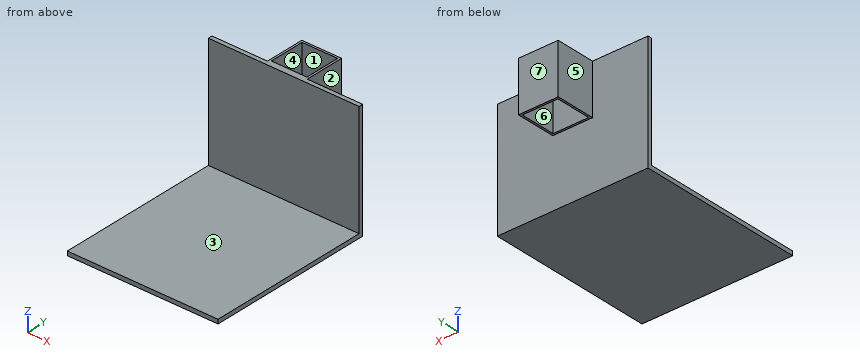
```python
from build123d import *

# Parameters (mm, degrees)
F0_W     = 60.325
F0_H     = 60.325
F0_W_2   = 53.975
F0_H_2   = 53.975
F1_DEPTH = 76.2
F3_DEPTH = 114.3


with BuildPart() as f1:
    # F0 (on Top) → F1 (new body)
    with BuildSketch(Plane.XY):
        Rectangle(F0_W, F0_H)
        Rectangle(F0_W_2, F0_H_2, mode=Mode.SUBTRACT)
    extrude(amount=F1_DEPTH)

    # F2 (on Right) → F3 (join, symmetric)
    with BuildSketch(Plane.YZ):
        Polygon((-30.1625, -101.6), (-30.1625, 76.2), (-36.5125, 76.2), (-36.5125, -95.25), (-284.1625, -95.25), (-284.1625, -101.6), align=None)
    extrude(amount=F3_DEPTH, both=True)


solid = f1.part
```
Check sheet for the modelled part. Datum: model origin and axes. Units: mm. Face numbers are marked on the shaded views. A direction names the side the tool comes from. Give positions to 0.01 mm unless a question says otherwise; leave off trailing zeros. Order: outer loops, then holes, each group sorted by start corner. A loop starts at its lowest first (then second) coordinate and runs counter-clockwise, first axis right, second up. Notation, with made-up numbers: M 23.25,81 L 68.25,81 A12 cw 68.25,94 Z; hole C -7,34 d2. An arc over 180 degrees is marked long. Answer in a Markdown table with one row per item. Add a question column.
Q1. Thickness scan on L1, parallel to X at y = -11.5, z = 14.5; L2, parallel to Y at x = -1, z = 1; L3, parallel to Z at x = 31.5, y = -67.5. Record the ranges inside material, lowest first.
Q2. Sectioned sample at A-A, the plane x = -6.5. Record the boundary of the cut face in (y, z), and give its area (3 significant figures).
Q3. Gauge pin test, flat ends, axial feed: pin 1 Ø16 at (y, z) = (-3.5, 33.5) entering from +X; pin 2 Ø1.5 at (x, z) = (83.5, 47.5) entering from -Y; pin 3 Ø2 at (y, z) = (-18.5, 16) entering from -X; pin 4 Ø18 at (x, y) = (6.5, -14.5) entering from -Z. Record the tip position at first contact, or that the pin passes through.
Q4. Sectioned sample at D-D, the plane x = 92.5. Record the boundary of the cut face in (y, z).
Q5. Access from +Z, -Z, +X, -X, +Y, -Y to the whole of each face (thin tool, end or side, straight path). Record for the marked faces 1, 2 and 3.
Q6. Release check for a two-part mould opening along Y. For the marked faces 4, 5, 6 and 7 record: released by +Y, released by -Y, zero draft, split by the parting line, or undercut.
Q7. Sectioned sample at C-C, the plane z = 36. Record the boundary of the cut face in (x, y), and give its area (3 significant figures).
Q8. Sectioned sample at B-B, the plane y = -12. Record the boundary of the cut face in (x, z).
Verdict:
| question | item | result |
|---|---|---|
| 1 | L1 | -30.16 to -26.99, 26.99 to 30.16 |
| 1 | L2 | -36.51 to -26.99, 26.99 to 30.16 |
| 1 | L3 | -101.6 to -95.25 |
| 2 | outline | M -284.16,-101.6 L -30.16,-101.6 L -30.16,0 L -26.99,0 L -26.99,76.2 L -36.51,76.2 L -36.51,-95.25 L -284.16,-95.25 Z; M 26.99,0 L 30.16,0 L 30.16,76.2 L 26.99,76.2 Z |
| 2 | area | 3,190 mm² |
| 3 | pin 1 | x = 30.16 |
| 3 | pin 2 | y = -36.51 |
| 3 | pin 3 | x = -30.16 |
| 3 | pin 4 | through |
| 4 | outline | M -284.16,-101.6 L -30.16,-101.6 L -30.16,76.2 L -36.51,76.2 L -36.51,-95.25 L -284.16,-95.25 Z |
| 5 | face 1 | +Z, -Z |
| 5 | face 2 | +Z, -Z, +X, +Y |
| 5 | face 3 | +Z, +X, -X, -Y |
| 6 | face 4 | undercut |
| 6 | face 5 | zero draft |
| 6 | face 6 | undercut |
| 6 | face 7 | released by +Y |
| 7 | outline | M -114.3,-36.51 L 114.3,-36.51 L 114.3,-30.16 L 30.16,-30.16 L 30.16,30.16 L -30.16,30.16 L -30.16,-30.16 L -114.3,-30.16 Z; hole M -26.99,-26.99 L 26.99,-26.99 L 26.99,26.99 L -26.99,26.99 Z |
| 7 | area | 2,180 mm² |
| 8 | outline | M -30.16,0 L -26.99,0 L -26.99,76.2 L -30.16,76.2 Z; M 26.99,0 L 30.16,0 L 30.16,76.2 L 26.99,76.2 Z |
